Solid Edge part; units mm, degrees
sketch "Sketch1" plane through (0, 0, 0) normal (0, 0, 1) x (1, 0, 0)
  circle A0 centre (0, 0) radius 25
extrude "Protrusion1" add sketch "Sketch1" along normal blind 70
sketch "Sketch2" plane through (0, 0, 0) normal (0, 0, -1) x (0, -1, 0)
  circle A0 centre (0, 20) radius 2.5
  circle A1 centre (17.3205, 10) radius 2.5
  circle A2 centre (17.3205, -10) radius 2.5
  circle A3 centre (0, -20) radius 2.5
  circle A4 centre (-17.3205, -10) radius 2.5
  circle A5 centre (-17.3205, 10) radius 2.5
extrude "ExtrudedCutout_1" cut sketch "Sketch2" against normal blind 12
sketch "Sketch3" plane through (0, 0, 0) normal (0, 0, -1) x (1, 0, 0)
  circle A0 centre (0, 0) radius 15
extrude "ExtrudedCutout_3" cut sketch "Sketch3" against normal blind 60
sketch "Sketch4" plane through (0, 0, 0) normal (0, 0, -1) x (0, -1, 0)
  circle A0 centre (0, 0) radius 15
extrude "ExtrudedCutout_4" cut sketch "Sketch4" against normal blind 70
sketch "Sketch5" plane through (0, 0, 0) normal (0, 0, -1) x (1, 0, 0)
  circle A0 centre (0, 0) radius 23.75
  circle A1 centre (0, 0) radius 25
extrude "Cutout1" cut sketch "Sketch5" against normal up to vertex (70 mm away)
Design review of the part built by this model. Coordinates are the model's own, in mm. A direction names the side the tool comes from. Give positions to 0.01 mm unless a question says otherwise; leave off trailing zeros. Write each loop counter-clockwise with the first axis right and the second up, starting at its lowest first coordinate (ties: lowest second). Pieces come first, ordered by that corner, then holes. Notation, with made-up numbers: M 18.5,82.25 L 52.5,82.25 A20 ccw 52.5,106.25 Z; hole C 8,0 d4. An arc over 180 degrees is marked long. Return JSON: item names as keys, results as strings. Group by question number.
Item 1: Wall thickness on line 1 along Y through (x, z) = (10, 5.25); line 2 along X through (y, z) = (-1, 7); line 3 along X through (y, z) = (-1.5, 6.5): over which ranges is each line inside the solid? List them lowest first.
Item 2: Clearance check with flat-ended pins moving along their axes: pin 1 Ø6 at (y, z) = (5.5, 17) entering from -X; pin 2 Ø10 at (x, z) = (14, 11.5) entering from +Y; pin 3 Ø1.5 at (x, y) = (-9, -16.5) entering from -Z. State where each tip first meets the part, or that it passes through.
Item 3: Tool access review of faces 4 (the flat face through (16, 0, 0)), 5 (the flat face through (-10, 17, 12)): name each direction out of +Z, -Z, +X, -X, +Y, -Y from which nothing blocks a thin tool from reaching the whole face with its end or side.
Item 4: Take a section at A-A (y = 0). Give the boundary of the cut face in (x, z).
Item 5: Take a section at C-C (x = 0). Give the boundary of the cut face in (y, z), plus the area to 4 significant figures.
Item 6: The part is to be moulded in two halves that separate along Y. For faces 1 (the flat face through (16, 0, 70)), 2 (the cylindrical face through (-5.149, 23.185, 34.51)), 3 (the cylindrical face through (13.922, -5.583, 34.51)), say which applies: pulls with the +Y half, pulls with the -Y half, needs draft (parallel to the pull), parting line crosses it, or undercut.
Item 7: Take a section at D-D (x = -10). Give the boundary of the cut face in (y, z).
Item 8: Take a section at B-B (z = 4). Give the boundary of the cut face in (x, y).
Return value:
{
 "1": {"line 1": "y = -21.54 to -19.82, -14.82 to -11.18, 11.18 to 14.82, 19.82 to 21.54", "line 2": "x = -23.73 to -22.29, -17.71 to -14.97, 14.97 to 17.71, 22.29 to 23.73", "line 3": "x = -23.7 to -22, -18 to -14.92, 14.92 to 18, 22 to 23.7"},
 "2": {"pin 1": "stops at x = -23.62", "pin 2": "stops at y = 21.98", "pin 3": "stops at z = 12"},
 "3": {"face 4": "-Z, +X, -X, +Y, -Y", "face 5": "-Z"},
 "4": {"outline": "M -23.75,0 L -22.5,0 L -22.5,12 L -17.5,12 L -17.5,0 L -15,0 L -15,70 L -23.75,70 Z; M 15,0 L 17.5,0 L 17.5,12 L 22.5,12 L 22.5,0 L 23.75,0 L 23.75,70 L 15,70 Z"},
 "5": {"outline": "M -23.75,0 L -15,0 L -15,70 L -23.75,70 Z; M 15,0 L 23.75,0 L 23.75,70 L 15,70 Z", "area": "1,225 mm2"},
 "6": {"face 1": "needs draft", "face 2": "parting line crosses it", "face 3": "undercut"},
 "7": {"outline": "M -21.54,0 L -19.82,0 L -19.82,12 L -14.82,12 L -14.82,0 L -11.18,0 L -11.18,70 L -21.54,70 Z; M 11.18,0 L 14.82,0 L 14.82,12 L 19.82,12 L 19.82,0 L 21.54,0 L 21.54,70 L 11.18,70 Z"},
 "8": {"outline": "C 0,0 d47.5; hole C -20,0 d5; hole C 0,0 d30; hole C -10,-17.32 d5; hole C -10,17.32 d5; hole C 10,-17.32 d5; hole C 10,17.32 d5; hole C 20,0 d5"}
}
